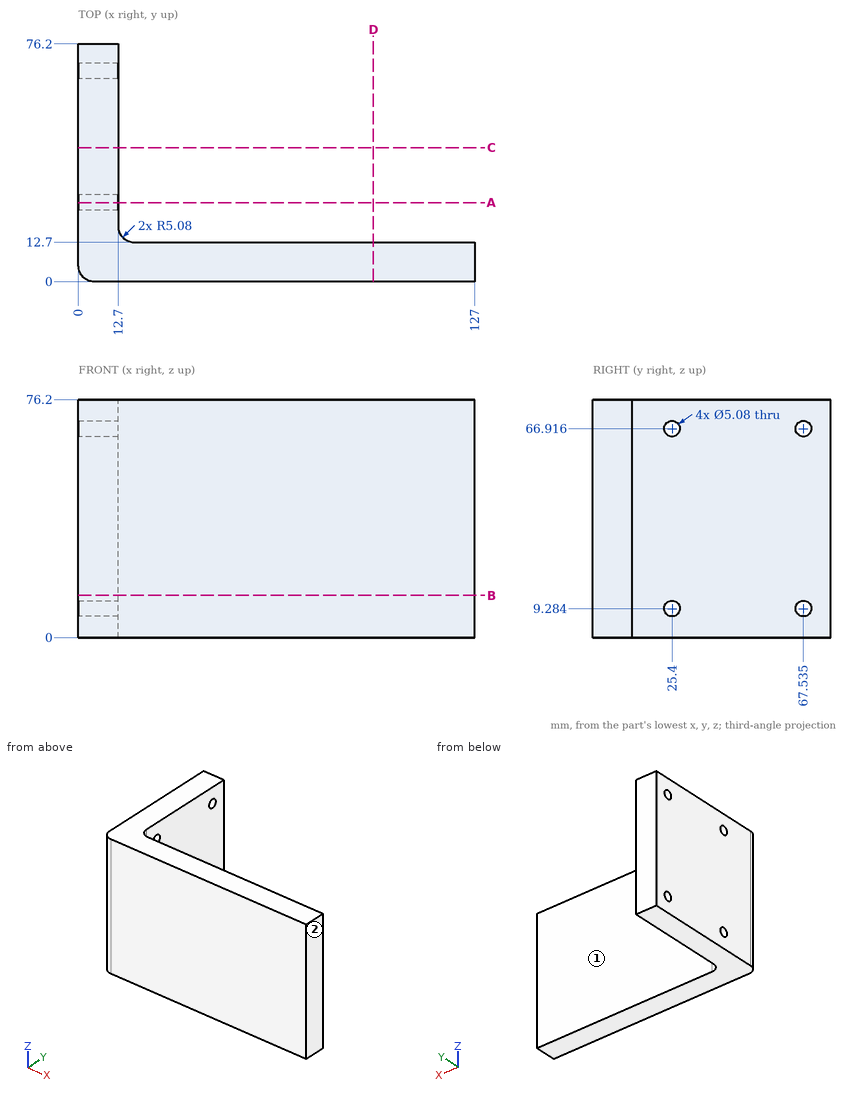
Study the drawing (mm; zero at the part's minimum x, y, z) and answer. A direction names the side the tool comes from. Give positions to 0.01 mm unless a question says otherwise; leave off trailing zeros. Loops run counter-clockwise (first coordinate to the right, second up) from the corner with the lowest first, then second, coordinate; pieces in that order, holes last. Notation, with made-up numbers: (66, 36.5) -> (72, 36.5) arc R5 ccw to (72, 41.5) -> close; hole circle Ø3 at (-25.75, -24). An arc over 180 degrees is marked (long way). Use a Markdown table: item, result. Add a question column.
1) Consider line 1 along Y through (x, z) = (63, 66); line 2 along X through (y, z) = (5, 71). Determine where each line is inside the solid, lowest interval first.
2) The part is cut by section B-B, the plane z = 13.5. Determine the outline of the cut face in (x, y), plus the area to 3 significant figures.
3) The part is cut by section A-A, the plane y = 25.4. Determine the outline of the cut face in (x, z) (1 decimal), plus the area to 3 significant figures.
4) The part is cut by section C-C, the plane y = 43. Determine the outline of the cut face in (x, z), plus the area to 3 significant figures.
5) Which of the six approach directions +Z, -Z, +X, -X, +Y, -Y give full straight-line access (tool end or side, diameter ignored) to the marked faces 1 and 2?
6) Each of these flat-tipped pins is pushed along its axis until it touches: P1, Ø12, axis at x = 35, z = 58.5, coming from the +Y side; P2, Ø8, axis at y = 25.4, z = 9.28, coming from the +X side. Where does it stop, or does it pass through?
Reported:
| question | item | result |
|---|---|---|
| 1 | line 1 | y = 0 to 12.7 |
| 1 | line 2 | x = 0 to 127 |
| 2 | outline | (0, 5.08) arc R5.08 ccw to (5.08, 0) -> (127, 0) -> (127, 12.7) -> (17.78, 12.7) arc R5.08 cw to (12.7, 17.78) -> (12.7, 76.2) -> (0, 76.2) -> close |
| 2 | area | 2,420 mm^2 |
| 3 | outline | (0, 0) -> (12.7, 0) -> (12.7, 6.7) -> (0, 6.7) -> close; (0, 11.8) -> (12.7, 11.8) -> (12.7, 64.4) -> (0, 64.4) -> close; (0, 69.5) -> (12.7, 69.5) -> (12.7, 76.2) -> (0, 76.2) -> close |
| 3 | area | 839 mm^2 |
| 4 | outline | (0, 0) -> (12.7, 0) -> (12.7, 76.2) -> (0, 76.2) -> close |
| 4 | area | 968 mm^2 |
| 5 | face 1 | +Z, -Z, +X, +Y |
| 5 | face 2 | +Z, -Z, +X, +Y, -Y |
| 6 | P1 | stops at y = 12.7 |
| 6 | P2 | stops at x = 12.7 |
